Source: CAD feature listing. Evaluate the final solid. Frame: model axes, mm. A direction names the side the tool comes from. Coordinates: 2 decimals unless noted, no trailing zeros. Order: outer loops, then holes, each group sorted by start corner. A loop starts at its lowest first (then second) coordinate and runs counter-clockwise, first axis right, second up. Notation, with made-up numbers: (-31.5, 61) -> (-12.5, 61) arc R20 cw to (-12.5, 74) -> close; hole circle Ø8 at (-17, 82.5). An arc over 180 degrees is marked (long way). Put each result on its own line as item: value.
from build123d import *
from OCP.BRepFilletAPI import BRepFilletAPI_MakeChamfer

# Parameters (mm, degrees)
EXTRUDE_1_DEPTH     = 17.5
CUT_EXTRUDE_1_DEPTH = 12.5
CUT_EXTRUDE_2_DEPTH = 135
CHAMFER_1_SIZE      = 1
CHAMFER_1_SIZE2     = 0.741639712
SKETCH_4_R          = 4.9
SKETCH_4_W          = 14.9
SKETCH_4_H          = 9.8
EXTRUDE_2_DEPTH     = 19.9
CHAMFER_2_SIZE      = 1
SKETCH_8_R          = 2
CUT_EXTRUDE_5_DEPTH = 141.031269382


with BuildPart() as part:
    # 스케치1 → 보스-돌출1 (new, symmetric)
    with BuildSketch(Plane.XY):
        Polygon((0, 0), (50, 0), (60.774208204, -2.663057759), (130.774208204, -2.663057759), (123.239760601, -17.169499956), (22.168183174, -27.799088209), (3.828389762, -35.803112621), (-1.495960418, -35.803112621), (0, -21.57), align=None)
    extrude(amount=EXTRUDE_1_DEPTH, both=True)

    # 스케치2 → 컷-돌출1 (cut, symmetric)
    with BuildSketch(Plane.XY):
        Polygon((0, 0), (0, -5.2), (34, -5.2), (34, -18.4), (42.1, -18.4), (42.1, 0), align=None)
    extrude(amount=CUT_EXTRUDE_1_DEPTH, both=True, mode=Mode.SUBTRACT)

    # 스케치3 → 컷-돌출2 (cut)
    with BuildSketch(Plane(origin=(0, 0, 0), x_dir=(0, 0, -1), z_dir=(1, 0, 0))):
        with BuildLine():
            Line((13.1, 0), (-13.1, 0))
            ThreePointArc((-13.1, 0), (0, -4.369440217), (13.1, 0))
        make_face()
    extrude(amount=CUT_EXTRUDE_2_DEPTH, mode=Mode.SUBTRACT)

    # 모따기1: one chamfer whose edges measure the first distance from different faces: ONE call of the kernel's chamfer builder (chamfer() names one face for all edges)
    chamfer_1_edges_1 = [part.edges().sort_by_distance(p)[0] for p in [
        (130.774208204, -2.663057759, 12.979729839),
    ]]
    chamfer_1_side_1 = [part.faces().sort_by_distance(p)[0] for p in [
        (126.871435624, -10.177257582, 0),
    ]]
    chamfer_1_edges_2 = [part.edges().sort_by_distance(p)[0] for p in [
        (95.774208204, -2.663057759, 17.5),
        (55.387104102, -1.331528879, 17.5),
        (25, 0, 17.5),
        (25, 0, -17.5),
        (55.387104102, -1.331528879, -17.5),
        (95.774208204, -2.663057759, -17.5),
    ]]
    chamfer_1 = BRepFilletAPI_MakeChamfer(part.part.solid().wrapped)
    for e in chamfer_1_edges_1:
        chamfer_1.Add(CHAMFER_1_SIZE, CHAMFER_1_SIZE2, e.wrapped, chamfer_1_side_1[0].wrapped)  # the first distance lies on this face
    for e in chamfer_1_edges_2:
        chamfer_1.Add(CHAMFER_1_SIZE, e.wrapped)
    add(Compound.cast(chamfer_1.Shape()), mode=Mode.REPLACE)

    # 스케치4 → 보스-돌출2 (add)
    with BuildSketch(Plane.ZY):
        with Locations(Location((10, -13.57, 0), (0, 0, 90))):
            Circle(SKETCH_4_R)
        with Locations(Location((-10, -13.57, 0), (0, 0, 90))):
            Circle(SKETCH_4_R)
        with Locations((0, -26.47)):
            Rectangle(SKETCH_4_W, SKETCH_4_H)
    extrude(amount=EXTRUDE_2_DEPTH)

    # 모따기2
    chamfer_2_edges = [part.edges().sort_by_distance(p)[0] for p in [
        (-19.9, -18.47, -10),
        (-19.9, -26.47, 7.45),
        (-19.9, -21.57, 0),
        (-19.9, -26.47, -7.45),
        (-19.9, -31.37, 0),
        (-19.9, -18.47, 10),
    ]]
    chamfer(chamfer_2_edges, length=CHAMFER_2_SIZE)

    # 스케치8 → 컷-돌출5 (cut, through all)
    with BuildSketch(Plane.XY.offset(17.5)):
        with Locations((38.05, -10.3)):
            Circle(SKETCH_8_R)
    extrude(amount=-CUT_EXTRUDE_5_DEPTH, mode=Mode.SUBTRACT)


solid = part.part
1. Ray query, line 1 along Y through (x, z) = (38, -15); line 2 along X through (y, z) = (-10, -15); line 3 along Y through (x, z) = (38, -13). Return the intervals inside material, ascending.
Numbers:
line 1: y = -26.13 to -12.3, -8.3 to 0
line 2: x = 0 to 36.07, 40.03 to 126.96
line 3: y = -26.13 to -12.3, -8.3 to -0.07
2. Cut plane C-C on x = 68.5. Output: boundary loops of the cut face in (y, z), plus the area to 3 significant figures.
Numbers:
outline: (-22.93, -17.5) -> (-3.66, -17.5) -> (-2.66, -16.5) -> (-2.66, -8.46) arc R21.82 cw to (-2.66, 8.46) -> (-2.66, 16.5) -> (-3.66, 17.5) -> (-22.93, 17.5) -> close
area: 689 mm2
3. First-contact query: pin 1 (3.5 mm diameter, centred on x = 38.05, y = -10.3, fed in from -Z); pin 2 (5 mm diameter, centred on y = -20.5, z = -13, fed in from -X); pin 3 (1.5 mm diameter, centred on x = 48.5, z = 13, fed in from -Y); pin 4 (4.5 mm diameter, centred on x = 38.05, y = -10.3, fed in from +Z). Flat tips, straight axial feed; report the tip coordinate or a pass-through.
Numbers:
pin 1: passes through
pin 2: stops at x = -0.15
pin 3: stops at y = -25.11
pin 4: stops at z = 17.5
4. Cut plane D-D on z = -1.5. Output: boundary loops of the cut face in (x, y), plus the area to 3 significant figures.
Numbers:
outline: (-19.9, -30.37) -> (-18.9, -31.37) -> (-1.03, -31.37) -> (-1.5, -35.8) -> (3.83, -35.8) -> (22.17, -27.8) -> (123.24, -17.17) -> (129.91, -4.32) -> (42.1, -4.32) -> (42.1, -18.4) -> (34, -18.4) -> (34, -5.2) -> (0, -5.2) -> (0, -21.57) -> (-18.9, -21.57) -> (-19.9, -22.57) -> close
area: 2,560 mm2
5. Pull-direction query (Z, two-part tool) for faces 5 (the flat face through (-9, -21.57, 0)), 6 (the flat face through (55.2, -1.8, -17)), 7 (the flat face through (34, -12, 0)), 8 (the flat face through (38, -18.4, 0)); classes: pulls with the +Z half, pulls with the -Z half, needs draft (parallel to the pull), parting line crosses it, or undercut.
Numbers:
face 5: needs draft
face 6: pulls with the -Z half
face 7: undercut
face 8: undercut
6. Set-up query: faces 1 (the flat face through (42.1, -12, 0)), 2 (the flat face through (95, -2.663, -12)), 3 (the flat face through (0, -13, 0)), 4 (the flat face through (17, -5.2, 0)). Return all of +Z, -Z, +X, -X, +Y, -Y with unobstructed straight access to the full face (end or side cutting, diameter ignored); none if empty.
Numbers:
face 1: +Y
face 2: +Z, -Z, +X, +Y
face 3: -X
face 4: -X, +Y
7. Cut plane B-B on z = -10. Output: boundary loops of the cut face in (x, y).
Numbers:
outline: (-19.9, -17.47) -> (-18.9, -18.47) -> (0, -18.47) -> (0, -21.57) -> (-1.5, -35.8) -> (3.83, -35.8) -> (22.17, -27.8) -> (123.24, -17.17) -> (130.77, -2.66) -> (60.77, -2.66) -> (57.86, -1.94) -> (42.1, -1.94) -> (42.1, -18.4) -> (34, -18.4) -> (34, -5.2) -> (0, -5.2) -> (0, -8.67) -> (-18.9, -8.67) -> (-19.9, -9.67) -> close
8. Cut plane A-A on x = 38.05. Output: boundary loops of the cut face in (y, z), plus the area to 3 significant figures.
Numbers:
outline: (-26.13, -17.5) -> (-12.3, -17.5) -> (-12.3, -12.5) -> (-18.4, -12.5) -> (-18.4, 12.5) -> (-12.3, 12.5) -> (-12.3, 17.5) -> (-26.13, 17.5) -> close; (-8.3, -17.5) -> (-1, -17.5) -> (0, -16.5) -> (0, -13.1) arc R21.82 cw to (-0.43, -12.5) -> (-8.3, -12.5) -> close; (-8.3, 12.5) -> (-0.43, 12.5) arc R21.82 cw to (0, 13.1) -> (0, 16.5) -> (-1, 17.5) -> (-8.3, 17.5) -> close
area: 413 mm2
